Input: part model. Units: mm. Frame: model coordinates. Face numbers are marked on the shaded views. A direction names the side the tool comes from. Coordinates: 2 decimals unless noted, no trailing zeros. Order: outer loops, then holes, each group sorted by start corner. A loop starts at its lowest first (then second) coordinate and runs counter-clockwise, first axis right, second up. Notation, with made-up numbers: M -39,58.25 L 11,58.25 A5 cw 11,62.25 Z; hole C -30,-17.75 d2. An arc over 180 degrees is marked long. One line per item, written item: value.
```python
from build123d import *

# Parameters (mm, degrees)
F0_R     = 44.45
F0_R_2   = 28.575
F1_DEPTH = 7.112
F2_R     = 3.81
F3_W     = 80.1546871662
F3_H     = 130.5045634508
F4_DEPTH = 12.7
F6_R     = 1.27
F7_DEPTH = 5.08
F5_R     = 1.27
F8_DEPTH = 6.35
F9_R     = 1.27


with BuildPart() as f1:
    # F0 (on Top) → F1 (new body)
    with BuildSketch(Plane.XY):
        Circle(F0_R)
        Circle(F0_R_2, mode=Mode.SUBTRACT)
    extrude(amount=F1_DEPTH)

    # F2
    f2_edges = [f1.edges().sort_by_distance(p)[0] for p in [
        (-44.45, 0, 7.112),
    ]]
    fillet(f2_edges, radius=F2_R)

    # F3 (on Top) → F4 (cut, symmetric)
    with BuildSketch(Plane.XY):
        with Locations((40.0773435831, -1.4468356967)):
            Rectangle(F3_W, F3_H)
    extrude(amount=F4_DEPTH, both=True, mode=Mode.SUBTRACT)

    # F6 (on face) → F7 (join)
    with BuildSketch(Plane.YZ):
        with Locations((35.56, 3.556)):
            Circle(F6_R)
    extrude(amount=F7_DEPTH)

    # F5 (on face) → F8 (cut)
    with BuildSketch(Plane.YZ):
        with Locations((-35.56, 3.302)):
            Circle(F5_R)
    extrude(amount=-F8_DEPTH, mode=Mode.SUBTRACT)

    # F9
    f9_edges = [f1.edges().sort_by_distance(p)[0] for p in [
        (5.08, 34.29, 3.556),
        (0, -36.83, 3.302),
    ]]
    fillet(f9_edges, radius=F9_R)


solid = f1.part
```
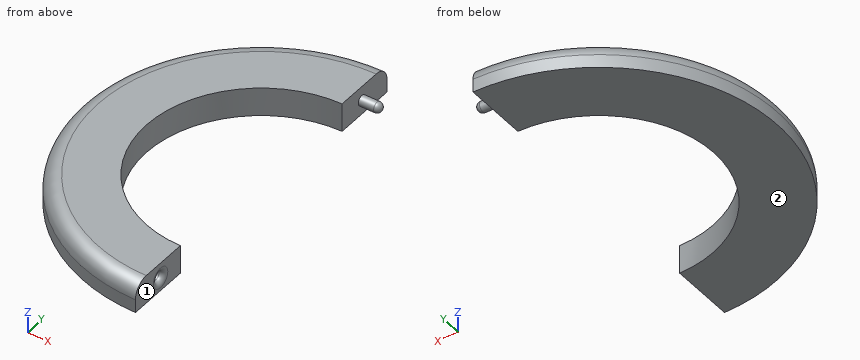
(1) Access query for the marked faces 1 and 2. Directions: +Z, -Z, +X, -X, +Y, -Y. A direction counts if a zero-diameter tool reaches every point of the face in a straight line with its end or side. Return the directions, or none.
Data:
face 1: +Z, -Z, +X, -Y
face 2: -Z, +X, -X, +Y, -Y
(2) Cut plane B-B on x = 1. Output: boundary loops of the cut face in (y, z).
Data:
outline: C 35.56,3.56 d2.54
(3) Cut plane A-A on y = 0. Output: boundary loops of the cut face in (x, z) (3 decimals), plus the area to 3 significant figures.
Data:
outline: M -44.45,0 L -28.575,0 L -28.575,7.112 L -40.64,7.112 A3.81 ccw -44.45,3.302 Z
area: 110 mm2
(4) First-contact query: pin 1 (3 mm diameter, centred on y = -35.56, z = 3.302, fed in from +X); pin 2 (3 mm diameter, centred on y = -35, z = 1.5, fed in from +X); pin 3 (3 mm diameter, centred on x = -27, z = 5, fed in from -Y). Flat tips, straight axial feed; report the tip coordinate or a pass-through.
Data:
pin 1: stops at x = -0.54
pin 2: stops at x = 0
pin 3: stops at y = -36.12
(5) Ray query, line 1 (Z direction, x = -2.6, y = -35.56); line 2 (Y direction, x = -7.5, z = 3); line 3 (Y direction, x = -25.5, z = 2.5). Return the intervals inside material, ascending. Write a range as from..to.
Data:
line 1: z = 0..2.03, 4.57..7.11
line 2: y = -43.81..-27.57, 27.57..43.81
line 3: y = -36.41..-12.89, 12.89..36.41
